```python
from build123d import *

# Parameters (mm, degrees)
PAD_DEPTH = 5
FILLET_R  = 2


with BuildPart() as part:
    # Sketch → Pad (new body)
    with BuildSketch(Plane.XY):
        with BuildLine():
            ThreePointArc((10.606602, -10.606602), (5.740251, 13.858193), (-15, 0))
            Line((-20, 0), (-15, 0))
            ThreePointArc((14.142136, -14.142136), (7.653669, 18.477591), (-20, 0))
            Line((14.142136, -14.142136), (-10.606602, -38.890873))
            ThreePointArc((-10.606602, -38.890873), (-5.740251, -63.355668), (15, -49.497475))
            Line((15, -49.497475), (20, -49.497475))
            ThreePointArc((-14.142136, -35.355339), (-7.653669, -67.975065), (20, -49.497475))
            Line((10.606602, -10.606602), (-14.142136, -35.355339))
        make_face()
    extrude(amount=PAD_DEPTH)

    # Fillet
    fillet_edges = [part.edges().sort_by_distance(p)[0] for p in [
        (-15, 0, 2.5),
        (-20, 0, 2.5),
        (20, -49.497475, 2.5),
        (15, -49.497475, 2.5),
    ]]
    fillet(fillet_edges, radius=FILLET_R)


solid = part.part
```
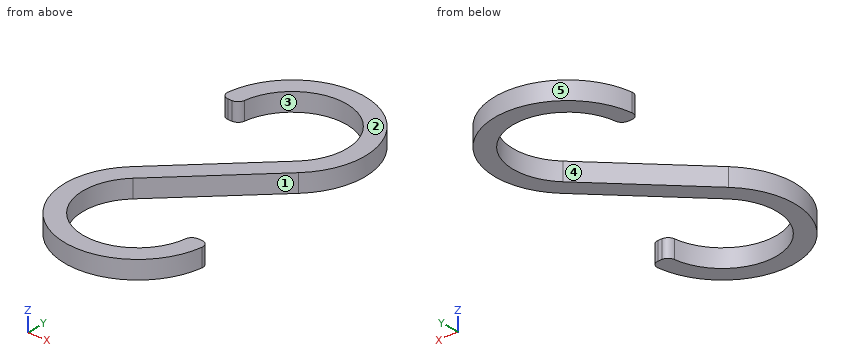
CAD build for the part. Positions are in the model's coordinates, mm. Face numbers are marked on the shaded views. A direction names the side the tool comes from. Give positions to 0.01 mm unless a question says otherwise; leave off trailing zeros. Order: outer loops, then holes, each group sorted by start corner. A loop starts at its lowest first (then second) coordinate and runs counter-clockwise, first axis right, second up. Notation, with made-up numbers: M -34.75,0 L -17.75,0 A11 cw -17.75,5 Z; hole C -4.5,-20 d8. An arc over 180 degrees is marked long. Put each result on its own line as item: value. Start each with the question number.
(1) Saw through at A-A, the plane y = -61. Write the cut outline in (x, z).
(2) Which spindle directions (+Z, -Z, +X, -X, +Y, -Y) get a long thin tool onto all of the face, cutting with end or side? Do the marked faces 4 and 5. Say none if no direction does.
(3) Saw through at D-D, the plane x = 8.5. Write the cut outline in (y, z), then the cut area to 3 significant figures.
(4) Mould opens along Y. For the marked faces 1, 2 and 3 say: +Y half, -Y half, draft (parallel to the pull), parting line (faces both ways), or undercut.
(5) Saw through at B-B, the plane z = 3.75. Write the cut outline in (x, y), then the cut area to 3 significant figures.
(6) Drill centre lines: line 1 along Y through (x, z) = (13.5, 3); line 2 along Y through (x, z) = (-3, 4.15); line 3 along Y through (x, z) = (-16, 4.6). Where is each one in solid material? Low to high.
(7) Flat gauge pins, fed straight in: pin 1 Ø1 at (x, z) = (-15, 1.5) entering from -Y; pin 2 Ø1.5 at (x, z) = (-4, 4.5) entering from +Y. Where does each tip first touch, or does it go through?
(8) Saw through at C-C, the plane x = 1.5. Write the cut outline in (y, z), then the cut area to 3 significant figures.
Check result:
1. outline: M -16.36,0 L -9.63,0 L -9.63,5 L -16.36,5 Z; M 9.63,0 L 16.36,0 L 16.36,5 L 9.63,5 Z
2. face 4: +Z, -Z, -X
2. face 5: +Z, -Z
3. outline: M -67.6,0 L -61.86,0 L -61.86,5 L -67.6,5 Z; M -19.78,0 L -12.71,0 L -12.71,5 L -19.78,5 Z; M 12.36,0 L 18.1,0 L 18.1,5 L 12.36,5 Z
3. area: 92.8 mm2
4. face 1: undercut
4. face 2: draft
4. face 3: undercut
5. outline: M -19.88,2.22 A2 ccw -17.89,0 L -16.88,0 A2 ccw -14.9,1.76 A15 cw long 10.61,-10.61 L -14.14,-35.36 A20 ccw long 19.88,-51.72 A2 ccw 17.89,-49.5 L 16.88,-49.5 A2 ccw 14.9,-51.26 A15 cw long -10.61,-38.89 L 14.14,-14.14 A20 ccw long Z
5. area: 859 mm2
6. line 1: y = -64.25 to -56.04, -14.78 to -6.54, 6.54 to 14.76
6. line 2: y = -69.27 to -64.19, -31.28 to -24.21, 14.7 to 19.77
6. line 3: y = -61.5 to -37.5, 0.2 to 12
7. pin 1: stops at y = -63.27
7. pin 2: stops at y = 19.73
8. outline: M -69.44,0 L -64.42,0 L -64.42,5 L -69.44,5 Z; M -26.78,0 L -19.71,0 L -19.71,5 L -26.78,5 Z; M 14.92,0 L 19.94,0 L 19.94,5 L 14.92,5 Z
8. area: 85.5 mm2
